from build123d import *
from build123d.topology import SkipClean

# Parameters (mm, degrees)
REVOLVE1_ANGLE     = 190
CUT_EXTRUDE1_DEPTH = 45.06204684


with BuildPart() as part:
    # Sketch1 → Revolve1 (revolve)
    with BuildSketch(Plane.XY):
        Polygon((15.897098368, 102.642966667), (5.2, 102.642966667), (5.2, 99.642966667), (12.897098368, 99.642966667), (12.897098368, 77.4), (9.725, 77.4), (9.725, 67.748), (2.7, 67.748), (2.7, 64.748), (15.897098368, 64.748), align=None)
    revolve(axis=Axis((0, 104.537715, 0), (0, -1, 0)), revolution_arc=REVOLVE1_ANGLE)

    # Sketch2 → Cut-Extrude1 (cut, through all)
    with SkipClean():  # the faces are left unmerged after this step: merging them gives an invalid solid
        with BuildSketch(Plane(origin=(0, 102.642966667, 0), x_dir=(1, 0, 0), z_dir=(0, 1, 0))):
            with BuildLine():
                Line((0, 0), (0, -12.897098368))
                ThreePointArc((0, -12.897098368), (1.002621368, -12.858067378), (1.999174193, -12.741210651))
                Line((1.999174193, -12.741210651), (1.999174193, 0))
                Line((1.999174193, 0), (0, 0))
            make_face()
        extrude(amount=-CUT_EXTRUDE1_DEPTH, mode=Mode.SUBTRACT)


solid = part.part
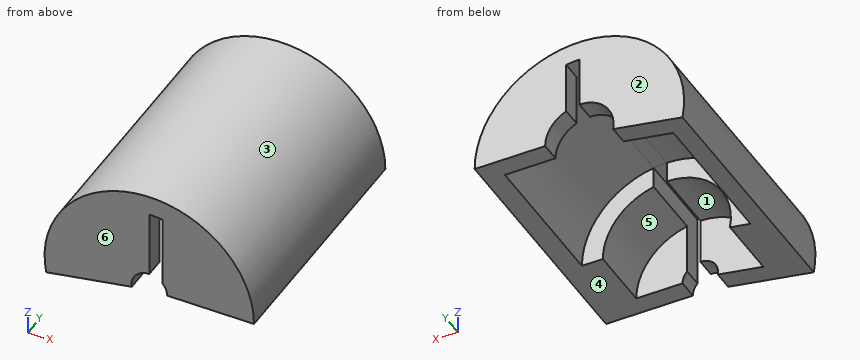
Can you work these out from the model? Positions are in its coordinate system, mm. Face numbers are marked on the shaded views. A direction names the side the tool comes from. Coordinates: 2 decimals unless noted, no trailing zeros. Loops run counter-clockwise (first coordinate to the right, second up) from the corner with the lowest first, then second, coordinate; pieces in that order, holes last. Notation, with made-up numbers: (89, 78.25) - (139, 78.25) arc R25 ccw to (139, 107.25) - close; hole circle Ø1 at (14.5, -32.75). An arc over 180 degrees is marked (long way). Put each result on its own line as item: value. Start each with the question number.
Item 1: Suppose I cut it at B-B (x = -11.5). Please give me the cut outline in (y, z).
Item 2: If we mould it in two halves opening along Y, with no side actions, what happens to the marked faces 1, 2 and 3? For each: +Y half, -Y half, draft (parallel to the pull), parting line (faces both ways), or undercut.
Item 3: Which directions (+Z, -Z, +X, -X, +Y, -Y) give clear straight access to the entire face, cutting with the end or side of a thin tool? Please do the marked faces 4, 5 and 6.
Item 4: If I drill on line 1 along Y through (x, z) = (5.5, 4.5); line 2 along X through (y, z) = (87, -0.5); line 3 along X through (y, z) = (96.5, 6.5), over which ranges is the centre line in solid material (lowest first)?
Item 5: Suppose I cut it at A-A (z = 2.25). Please give me the cut outline in (x, y).
Item 6: Suppose I cut it at D-D (z = 6.25). Please give me the cut outline in (x, y), and give its area (3 significant figures).
Item 7: For pin 1 (2.5 mm diameter, centred on y = 101.5, z = 9.5, fed in from -X); pin 2 (1 mm diameter, centred on y = 93.5, z = 12, fed in from +X); pin 3 (1.5 mm diameter, centred on y = 101.5, z = 9.5, fed in from +X), each with a flat end and sliding along its axis, tell me the tip position at first contact or that it passes through.
Here are the results:
1. outline: (64.75, -2.03) - (77.4, -2.03) - (77.4, 5.84) - (99.64, 5.84) - (99.64, -2.03) - (102.64, -2.03) - (102.64, 10.98) - (64.75, 10.98) - close
2. face 1: undercut
2. face 2: +Y half
2. face 3: draft
3. face 4: -Z, +X, +Y, -Y
3. face 5: -Z
3. face 6: +Z, -Z, +X, -X, -Y
4. line 1: 64.75 to 67.75, 99.64 to 102.64
4. line 2: -15.89 to -12.89
4. line 3: -14.51 to -11.14, 11.14 to 14.51
5. outline: (-15.74, 64.75) - (-1.49, 64.75) - (-1.49, 67.75) - (-9.46, 67.75) - (-9.46, 77.4) - (-12.7, 77.4) - (-12.7, 99.64) - (-4.69, 99.64) - (-4.69, 102.64) - (-15.74, 102.64) - close; (2, 64.75) - (15.74, 64.75) - (15.74, 102.64) - (4.69, 102.64) - (4.69, 99.64) - (12.7, 99.64) - (12.7, 77.4) - (9.46, 77.4) - (9.46, 67.75) - (2, 67.75) - close
6. outline: (-14.62, 64.75) - (0, 64.75) - (0, 67.75) - (-7.45, 67.75) - (-7.45, 77.4) - (-11.28, 77.4) - (-11.28, 99.64) - (0, 99.64) - (0, 102.64) - (-14.62, 102.64) - close; (2, 64.75) - (14.62, 64.75) - (14.62, 102.64) - (2, 102.64) - (2, 99.64) - (11.28, 99.64) - (11.28, 77.4) - (7.45, 77.4) - (7.45, 67.75) - (2, 67.75) - close
6. area: 450 mm²
7. pin 1: x = -13.59
7. pin 2: x = 10.98
7. pin 3: x = 13.27
